The listing builds one solid part. Answer for the finished solid, in the listing's coordinates (mm). A direction names the side the tool comes from. Round coordinates to 2 decimals unless told otherwise and drop trailing zeros. Loops run counter-clockwise (first coordinate to the right, second up) from the corner with the lowest first, then second, coordinate; pieces in that order, holes last. Notation, with made-up numbers: (48.5, 74) -> (99.5, 74) arc R11 cw to (99.5, 87) -> close; hole circle Ø9 at (-40, 71.5). An arc over 180 degrees is marked (long way). Use a Markdown table: item, result. Add a question column.
Q1. Section C-C on z = -24.5 is taken. Give the vertices of the cut face in (x, y), then the cut area to 3 significant figures.
Q2. For a pull along Z with two mould halves and no side action, classify faces 4 (the flat face through (5, -20, -50)), 5 (the flat face through (4, -36.2, 27)), 6 (the flat face through (5, -26, -40)), 7 (the cylindrical face through (4.93, -40.059, 23.403)) as released by +Z, released by -Z, zero draft, split by the parting line, or undercut.
Q3. Which of the six approach directions +Z, -Z, +X, -X, +Y, -Y give full straight-line access (tool end or side, diameter ignored) to faces 1 (the cylindrical face through (4.93, -39.997, -41.141)), 2 (the flat face through (5, -41.2, -45)), 3 (the flat face through (4, -28.8, 27))?
Q4. Section B-B on x = 3.75 is taken. Give the number of separate pieces and of enclosed holes in the cut face, then the cut area to 3 significant figures.
Q5. Given pin 1 Ø1.5 at (x, z) = (3.5, -15.5) entering from +Y; pin 2 Ø6 at (x, y) = (8, -5.5) entering from +Z; pin 3 Ø2 at (y, z) = (-32, -43) entering from -X, each flat-ended and moving along its own axis, determine where each tip first touches the part or whether it passes through.
Q6. Consider line 1 (Z direction, x = 1.25, y = -27); line 2 (Y direction, x = 7.5, z = -13.8) (3 decimals); line 3 (Y direction, x = 2.75, z = 11). Determine where each line is inside the solid, lowest interval first.
Q7. Section A-A on y = -22.5 is taken. Give the vertices of the cut face in (x, z).
from build123d import *

# Parameters (mm, degrees)
BOSS_EXTRUDE1_DEPTH = 10
SKETCH3_R           = 2.055
CUT_EXTRUDE1_DEPTH  = 11
SKETCH5_W           = 10
SKETCH5_H           = 13.8
BOSS_EXTRUDE2_DEPTH = 10
SKETCH10_W          = 10
SKETCH10_H          = 7.4
BOSS_EXTRUDE5_DEPTH = 2.52893219
SKETCH11_W          = 10
SKETCH11_H          = 5
BOSS_EXTRUDE6_DEPTH = 10
FILLET1_R           = 4
FILLET2_R           = 4
FILLET3_R           = 4


with BuildPart() as part:
    # Sketch1 → Boss-Extrude1 (new body)
    with BuildSketch(Plane(origin=(0, 0, 0), x_dir=(0, 0, -1), z_dir=(1, 0, 0))):
        Polygon((17.8, -5), (50, -5), (50, -15), (-32.2, -15), (-32.2, -5), (0, -5), (0, 0), (17.8, 0), align=None)
    extrude(amount=BOSS_EXTRUDE1_DEPTH)

    # Sketch3 → Cut-Extrude1 (cut, through all)
    with BuildSketch(Plane(origin=(10, 0, 0), x_dir=(0, 0, -1), z_dir=(1, 0, 0))):
        with Locations((4, -4)):
            Circle(SKETCH3_R)
        with Locations((13.8, -4)):
            Circle(SKETCH3_R)
    extrude(amount=-CUT_EXTRUDE1_DEPTH, mode=Mode.SUBTRACT)

    # Sketch5 → Boss-Extrude2 (add)
    with BuildSketch(Plane(origin=(10, 0, 0), x_dir=(0, 0, -1), z_dir=(1, 0, 0))):
        with Locations((-27.2, -21.9)):
            Rectangle(SKETCH5_W, SKETCH5_H)
        with Locations((45, -21.9)):
            Rectangle(SKETCH5_W, SKETCH5_H)
    extrude(amount=-BOSS_EXTRUDE2_DEPTH)

    # Sketch10 → Boss-Extrude5 (add)
    with BuildSketch(Plane(origin=(10, 0, 0), x_dir=(0, 0, -1), z_dir=(1, 0, 0))):
        with Locations((-27.2, -32.5)):
            Rectangle(SKETCH10_W, SKETCH10_H)
    boss_extrude5 = extrude(amount=-BOSS_EXTRUDE5_DEPTH)

    # Sketch11 → Boss-Extrude6 (add)
    with BuildSketch(Plane(origin=(10, 0, 0), x_dir=(0, 0, -1), z_dir=(1, 0, 0))):
        with Locations((-27.2, -38.7)):
            Rectangle(SKETCH11_W, SKETCH11_H)
    boss_extrude6 = extrude(amount=-BOSS_EXTRUDE6_DEPTH)

    # Mirror1: Boss-Extrude5, Boss-Extrude6 across plane
    add(boss_extrude5.mirror(Plane.XY.offset(-8.9)))
    add(boss_extrude6.mirror(Plane.XY.offset(-8.9)))

    # Fillet1
    fillet1_edges = [part.edges().sort_by_distance(p)[0] for p in [
        (5, 0, 0),
        (5, 0, -17.8),
    ]]
    fillet(fillet1_edges, radius=FILLET1_R)

    # Fillet2
    fillet2_edges = [part.edges().sort_by_distance(p)[0] for p in [
        (5, -41.2, -50),
        (5, -41.2, -40),
        (5, -5, -50),
        (5, -5, 32.2),
        (5, -15, 22.2),
        (5, -15, -40),
        (5, -41.2, 22.2),
        (5, -41.2, 32.2),
    ]]
    fillet(fillet2_edges, radius=FILLET2_R)

    # Fillet3
    fillet3_edges = [part.edges().sort_by_distance(p)[0] for p in [
        (5, -5, -17.8),
        (5, -5, 0),
    ]]
    fillet(fillet3_edges, radius=FILLET3_R)


solid = part.part
Checked values:
| question | item | result |
|---|---|---|
| 1 | outline | (0, -15) -> (10, -15) -> (10, -5) -> (0, -5) -> close |
| 1 | area | 100 mm2 |
| 2 | face 4 | released by -Z |
| 2 | face 5 | zero draft |
| 2 | face 6 | undercut |
| 2 | face 7 | undercut |
| 3 | face 1 | +X, -X, -Y |
| 3 | face 2 | +Z, -Z, +X, -X, -Y |
| 3 | face 3 | +Z, -Z, -X |
| 4 | separate pieces | 3 |
| 4 | enclosed holes | 2 |
| 4 | area | 1,240 mm2 |
| 5 | pin 1 | stops at y = -0.11 |
| 5 | pin 2 | stops at z = 32.17 |
| 5 | pin 3 | stops at x = 7.47 |
| 6 | line 1 | z = -50 to -40, 22.2 to 32.2 |
| 6 | line 2 | y = -15 to -6.055, -1.945 to 0 |
| 6 | line 3 | y = -15 to -5 |
| 7 | outline | (0, -50) -> (10, -50) -> (10, -40) -> (0, -40) -> close; (0, 22.2) -> (10, 22.2) -> (10, 32.2) -> (0, 32.2) -> close |
